Verification items for the finished model (mm, model axes). A direction names the side the tool comes from. Coordinates: 2 decimals unless noted, no trailing zeros. Order: outer loops, then holes, each group sorted by start corner. A loop starts at its lowest first (then second) coordinate and runs counter-clockwise, first axis right, second up. Notation, with made-up numbers: (-10.75, 47.25) - (26.25, 47.25) arc R19 cw to (26.25, 62.25) - close; hole circle Ø1 at (46.5, -25.75). An arc over 180 degrees is marked (long way). One line per question, with ' | ' between items. Start each with the question number.
from build123d import *

# Parameters (mm, degrees)
SKETCH1_R                                       = 30
BOSS_EXTRUDE1_DEPTH                             = 5
CSK_FOR_M3_FLAT_HEAD_MACHINE_SCREW1_D           = 3.4
CSK_FOR_M3_FLAT_HEAD_MACHINE_SCREW1_CSINK_D     = 6.3
CSK_FOR_M3_FLAT_HEAD_MACHINE_SCREW1_CSINK_ANGLE = 90
CUT_EXTRUDE1_REACH                              = 44.72
SKETCH4_R                                       = 1.1
CUT_EXTRUDE2_REACH                              = 44.72
SKETCH5_R                                       = 5
SKETCH7_R                                       = 2
CUT_EXTRUDE3_DEPTH                              = 2.2
CUT_EXTRUDE4_DEPTH                              = 3
SKETCH9_R                                       = 1.7
CUT_EXTRUDE5_DEPTH                              = 43.720018727


with BuildPart() as part:
    # Sketch1 → Boss-Extrude1 (new body)
    with BuildSketch(Plane(origin=(0, 0, 0), x_dir=(1, 0, 0), z_dir=(0, 1, 0))):
        with Locations(Location((0, 0, 0), (0, 0, 270))):
            Circle(SKETCH1_R)
    extrude(amount=BOSS_EXTRUDE1_DEPTH)

    # CSK for M3 Flat Head Machine Screw1 (through all)
    with Locations(Plane(origin=(0, 5, 0), x_dir=(1, 0, 0), z_dir=(0, 1, 0))):
        with Locations((-15.5, -15.5), (15.5, 15.5), (-15.5, 15.5), (15.5, -15.5)):
            CounterSinkHole(CSK_FOR_M3_FLAT_HEAD_MACHINE_SCREW1_D / 2, CSK_FOR_M3_FLAT_HEAD_MACHINE_SCREW1_CSINK_D / 2, counter_sink_angle=CSK_FOR_M3_FLAT_HEAD_MACHINE_SCREW1_CSINK_ANGLE)

    # Sketch4 → Cut-Extrude1 (cut, up to next)
    with BuildSketch(Plane(origin=(0, 5, 0), x_dir=(1, 0, 0), z_dir=(0, 1, 0)), mode=Mode.PRIVATE) as cut_extrude1_sk1:
        with Locations(Location((-13.75, 23.815698604, 0), (0, 0, 270))):
            Circle(SKETCH4_R)
    cut_extrude1_tool1 = extrude(cut_extrude1_sk1.sketch, amount=-CUT_EXTRUDE1_REACH, mode=Mode.PRIVATE) & part.part
    # Sketch4 → Cut-Extrude1 (cut, up to next)
    with BuildSketch(Plane(origin=(0, 5, 0), x_dir=(1, 0, 0), z_dir=(0, 1, 0)), mode=Mode.PRIVATE) as cut_extrude1_sk2:
        with Locations(Location((-23.815698604, 13.75, 0), (0, 0, 270))):
            Circle(SKETCH4_R)
    cut_extrude1_tool2 = extrude(cut_extrude1_sk2.sketch, amount=-CUT_EXTRUDE1_REACH, mode=Mode.PRIVATE) & part.part
    # Sketch4 → Cut-Extrude1 (cut, up to next)
    with BuildSketch(Plane(origin=(0, 5, 0), x_dir=(1, 0, 0), z_dir=(0, 1, 0)), mode=Mode.PRIVATE) as cut_extrude1_sk3:
        with Locations(Location((13.75, 23.815698604, 0), (0, 0, 270))):
            Circle(SKETCH4_R)
    cut_extrude1_tool3 = extrude(cut_extrude1_sk3.sketch, amount=-CUT_EXTRUDE1_REACH, mode=Mode.PRIVATE) & part.part
    # Sketch4 → Cut-Extrude1 (cut, up to next)
    with BuildSketch(Plane(origin=(0, 5, 0), x_dir=(1, 0, 0), z_dir=(0, 1, 0)), mode=Mode.PRIVATE) as cut_extrude1_sk4:
        with Locations(Location((23.815698604, 13.75, 0), (0, 0, 270))):
            Circle(SKETCH4_R)
    cut_extrude1_tool4 = extrude(cut_extrude1_sk4.sketch, amount=-CUT_EXTRUDE1_REACH, mode=Mode.PRIVATE) & part.part
    # Sketch4 → Cut-Extrude1 (cut, up to next)
    with BuildSketch(Plane(origin=(0, 5, 0), x_dir=(1, 0, 0), z_dir=(0, 1, 0)), mode=Mode.PRIVATE) as cut_extrude1_sk5:
        with Locations(Location((23.815698604, -13.75, 0), (0, 0, 270))):
            Circle(SKETCH4_R)
    cut_extrude1_tool5 = extrude(cut_extrude1_sk5.sketch, amount=-CUT_EXTRUDE1_REACH, mode=Mode.PRIVATE) & part.part
    # Sketch4 → Cut-Extrude1 (cut, up to next)
    with BuildSketch(Plane(origin=(0, 5, 0), x_dir=(1, 0, 0), z_dir=(0, 1, 0)), mode=Mode.PRIVATE) as cut_extrude1_sk6:
        with Locations(Location((13.75, -23.815698604, 0), (0, 0, 270))):
            Circle(SKETCH4_R)
    cut_extrude1_tool6 = extrude(cut_extrude1_sk6.sketch, amount=-CUT_EXTRUDE1_REACH, mode=Mode.PRIVATE) & part.part
    # Sketch4 → Cut-Extrude1 (cut, up to next)
    with BuildSketch(Plane(origin=(0, 5, 0), x_dir=(1, 0, 0), z_dir=(0, 1, 0)), mode=Mode.PRIVATE) as cut_extrude1_sk7:
        with Locations(Location((-13.75, -23.815698604, 0), (0, 0, 270))):
            Circle(SKETCH4_R)
    cut_extrude1_tool7 = extrude(cut_extrude1_sk7.sketch, amount=-CUT_EXTRUDE1_REACH, mode=Mode.PRIVATE) & part.part
    # Sketch4 → Cut-Extrude1 (cut, up to next)
    with BuildSketch(Plane(origin=(0, 5, 0), x_dir=(1, 0, 0), z_dir=(0, 1, 0)), mode=Mode.PRIVATE) as cut_extrude1_sk8:
        with Locations(Location((-23.815698604, -13.75, 0), (0, 0, 270))):
            Circle(SKETCH4_R)
    cut_extrude1_tool8 = extrude(cut_extrude1_sk8.sketch, amount=-CUT_EXTRUDE1_REACH, mode=Mode.PRIVATE) & part.part
    add(cut_extrude1_tool1.solids().sort_by_distance((-13.75, 5, -23.815699))[0], mode=Mode.SUBTRACT)
    add(cut_extrude1_tool2.solids().sort_by_distance((-23.815699, 5, -13.75))[0], mode=Mode.SUBTRACT)
    add(cut_extrude1_tool3.solids().sort_by_distance((13.75, 5, -23.815699))[0], mode=Mode.SUBTRACT)
    add(cut_extrude1_tool4.solids().sort_by_distance((23.815699, 5, -13.75))[0], mode=Mode.SUBTRACT)
    add(cut_extrude1_tool5.solids().sort_by_distance((23.815699, 5, 13.75))[0], mode=Mode.SUBTRACT)
    add(cut_extrude1_tool6.solids().sort_by_distance((13.75, 5, 23.815699))[0], mode=Mode.SUBTRACT)
    add(cut_extrude1_tool7.solids().sort_by_distance((-13.75, 5, 23.815699))[0], mode=Mode.SUBTRACT)
    add(cut_extrude1_tool8.solids().sort_by_distance((-23.815699, 5, 13.75))[0], mode=Mode.SUBTRACT)

    # Sketch5 → Cut-Extrude2 (cut, up to next)
    with BuildSketch(Plane(origin=(0, 5, 0), x_dir=(1, 0, 0), z_dir=(0, 1, 0)), mode=Mode.PRIVATE) as cut_extrude2_sk1:
        with Locations(Location((0, 0, 0), (0, 0, 270))):
            Circle(SKETCH5_R)
    cut_extrude2_tool1 = extrude(cut_extrude2_sk1.sketch, amount=-CUT_EXTRUDE2_REACH, mode=Mode.PRIVATE) & part.part
    add(cut_extrude2_tool1.solids().sort_by_distance((0, 5, 0))[0], mode=Mode.SUBTRACT)

    # Sketch7 → Cut-Extrude3 (cut)
    with BuildSketch(Plane(origin=(0, 5, 0), x_dir=(1, 0, 0), z_dir=(0, 1, 0))):
        with Locations(Location((-13.75, 23.815698604, 0), (0, 0, 270))):
            Circle(SKETCH7_R)
        with Locations(Location((-23.815698604, 13.75, 0), (0, 0, 270))):
            Circle(SKETCH7_R)
        with Locations(Location((13.75, 23.815698604, 0), (0, 0, 270))):
            Circle(SKETCH7_R)
        with Locations(Location((23.815698604, 13.75, 0), (0, 0, 270))):
            Circle(SKETCH7_R)
        with Locations(Location((23.815698604, -13.75, 0), (0, 0, 270))):
            Circle(SKETCH7_R)
        with Locations(Location((13.75, -23.815698604, 0), (0, 0, 270))):
            Circle(SKETCH7_R)
        with Locations(Location((-13.75, -23.815698604, 0), (0, 0, 270))):
            Circle(SKETCH7_R)
        with Locations(Location((-23.815698604, -13.75, 0), (0, 0, 270))):
            Circle(SKETCH7_R)
    extrude(amount=-CUT_EXTRUDE3_DEPTH, mode=Mode.SUBTRACT)

    # Sketch8 → Cut-Extrude4 (cut)
    with BuildSketch(Plane(origin=(0, 0, 0), x_dir=(1, 0, 0), z_dir=(0, 1, 0))):
        Polygon((-9.08771324, 15.740381057), (-10.675426481, 12.990381057), (-9.08771324, 10.240381057), (-5.91228676, 10.240381057), (-4.324573519, 12.990381057), (-5.91228676, 15.740381057), align=None)
        Polygon((-18.175426481, 0), (-16.58771324, -2.75), (-13.41228676, -2.75), (-11.824573519, 0), (-13.41228676, 2.75), (-16.58771324, 2.75), align=None)
        Polygon((9.08771324, 15.740381057), (5.91228676, 15.740381057), (4.324573519, 12.990381057), (5.91228676, 10.240381057), (9.08771324, 10.240381057), (10.675426481, 12.990381057), align=None)
        Polygon((18.175426481, 0), (16.58771324, 2.75), (13.41228676, 2.75), (11.824573519, 0), (13.41228676, -2.75), (16.58771324, -2.75), align=None)
        Polygon((9.08771324, -15.740381057), (10.675426481, -12.990381057), (9.08771324, -10.240381057), (5.91228676, -10.240381057), (4.324573519, -12.990381057), (5.91228676, -15.740381057), align=None)
        Polygon((-9.08771324, -15.740381057), (-5.91228676, -15.740381057), (-4.324573519, -12.990381057), (-5.91228676, -10.240381057), (-9.08771324, -10.240381057), (-10.675426481, -12.990381057), align=None)
    extrude(amount=CUT_EXTRUDE4_DEPTH, mode=Mode.SUBTRACT)

    # Sketch9 → Cut-Extrude5 (cut, through all)
    with BuildSketch(Plane.XZ):
        with Locations(Location((15, 0, 0), (0, 0, 270))):
            Circle(SKETCH9_R)
        with Locations(Location((7.5, -12.990381057, 0), (0, 0, 270))):
            Circle(SKETCH9_R)
        with Locations(Location((-7.5, -12.990381057, 0), (0, 0, 270))):
            Circle(SKETCH9_R)
        with Locations(Location((-15, 0, 0), (0, 0, 270))):
            Circle(SKETCH9_R)
        with Locations(Location((-7.5, 12.990381057, 0), (0, 0, 270))):
            Circle(SKETCH9_R)
        with Locations(Location((7.5, 12.990381057, 0), (0, 0, 270))):
            Circle(SKETCH9_R)
    extrude(amount=-CUT_EXTRUDE5_DEPTH, mode=Mode.SUBTRACT)


solid = part.part
Item 1: Set-up check for faces 1 (the cylindrical face through (-22.725, 1.42, 13.607)), 2 (the flat face through (-9.89, 1.48, -11.63)), 3 (the cylindrical face through (-25.77, 3.92, 13.32)): record each of +Z, -Z, +X, -X, +Y, -Y from which the full face is reachable in a straight line by a thin tool's end or side.
Item 2: Thickness scan on probe 1 along X at (y, z) = (4.55, -17.5); probe 2 along X at (y, z) = (0.35, 12); probe 3 along X at (y, z) = (3.7, -15.5). Record the ranges inside material, lowest first. Write a range as from..to.
Item 3: Section check C-C (z = -16.5). Give the number of separate pieces and of enclosed holes in the cut face, then the cut area to 3 significant figures.
Item 4: Section check B-B (x = 7.5). Record the cut outline in (y, z).
Item 5: Section check A-A (x = 0). Record the cut outline in (y, z), then the cut area to 3 significant figures.
Item 6: Gauge pin test, flat ends, axial feed: pin 1 (1.2 mm diameter, centred on x = 14.5, z = 24, fed in from +Y); pin 2 (2.5 mm diameter, centred on x = 7, y = 2, fed in from +Z); pin 3 (4.5 mm diameter, centred on x = -15.5, z = -15.5, fed in from +Y); pin 4 (1.3 mm diameter, centred on x = -23.82, z = 13.75, fed in from +Y). Record the tip position at first contact, or that the pin passes through.
Completed:
1) face 1: +Y, -Y | face 2: -Y | face 3: +Y
2) probe 1: x = -24.37..-17.31, -13.69..13.69, 17.31..24.37 | probe 2: x = -27.5..-10.1, -4.9..4.9, 10.1..27.5 | probe 3: x = -25.69..-24.78, -22.85..-17.35, -13.65..13.65, 17.35..22.85, 24.78..25.69
3) separate pieces: 3 | enclosed holes: 0 | area: 218 mm^2
4) outline: (0, -29.05) - (5, -29.05) - (5, -14.69) - (3, -14.69) - (3, -15.74) - (0, -15.74) - close; (0, -10.24) - (3, -10.24) - (3, -11.29) - (5, -11.29) - (5, 11.29) - (3, 11.29) - (3, 10.24) - (0, 10.24) - close; (0, 15.74) - (3, 15.74) - (3, 14.69) - (5, 14.69) - (5, 29.05) - (0, 29.05) - close
5) outline: (0, -30) - (5, -30) - (5, -5) - (0, -5) - close; (0, 5) - (5, 5) - (5, 30) - (0, 30) - close | area: 250 mm^2
6) pin 1: stops at y = 2.8 | pin 2: stops at z = 29.44 | pin 3: stops at y = 4.1 | pin 4: passes through
